The model under review builds one solid part; all positions refer to its coordinate system, in mm. Coordinates: 2 decimals unless noted, no trailing zeros. Order: outer loops, then holes, each group sorted by start corner. A loop starts at its lowest first (then second) coordinate and runs counter-clockwise, first axis right, second up. Notation, with made-up numbers: (-23, -0.75) - (-7, -0.75) arc R11 ccw to (-7, 8.25) - close; hole circle Ø4 at (-10, 31). An arc over 180 degrees is marked (long way). Answer in a Markdown table with one row per item.
```python
from build123d import *

# Parameters (mm, degrees)
F0_W     = 54
F0_H     = 48
F0_R     = 1.5
F1_DEPTH = 3
F2_R     = 1.5
F3_DEPTH = 2


with BuildPart() as f1:
    # F0 (on Front) → F1 (new body)
    with BuildSketch(Plane.XZ):
        Rectangle(F0_W, F0_H)
        with Locations((-23, -20)):
            Circle(F0_R, mode=Mode.SUBTRACT)
        with Locations((-18, -15)):
            Circle(F0_R, mode=Mode.SUBTRACT)
        with Locations((23, -20)):
            Circle(F0_R, mode=Mode.SUBTRACT)
        with Locations((18, -15)):
            Circle(F0_R, mode=Mode.SUBTRACT)
        with Locations((-18, 15)):
            Circle(F0_R, mode=Mode.SUBTRACT)
        with Locations((-23, 20)):
            Circle(F0_R, mode=Mode.SUBTRACT)
        with Locations((18, 15)):
            Circle(F0_R, mode=Mode.SUBTRACT)
        with Locations((23, 20)):
            Circle(F0_R, mode=Mode.SUBTRACT)
    extrude(amount=F1_DEPTH)

    # F2 (on face) → F3 (cut)
    with BuildSketch(Plane.XZ.offset(3)):
        Polygon((-25.6, -18.498889), (-25.6, -21.501111), (-23, -23.002221), (-20.4, -21.501111), (-20.4, -18.498889), (-23, -16.997779), align=None)
        with Locations((-23, -20)):
            Circle(F2_R, mode=Mode.SUBTRACT)
        Polygon((23, -16.997779), (20.4, -18.498889), (20.4, -21.501111), (23, -23.002221), (25.6, -21.501111), (25.6, -18.498889), align=None)
        with Locations((23, -20)):
            Circle(F2_R, mode=Mode.SUBTRACT)
        Polygon((-25.6, 21.501111), (-25.6, 18.498889), (-23, 16.997779), (-20.4, 18.498889), (-20.4, 21.501111), (-23, 23.002221), align=None)
        with Locations((-23, 20)):
            Circle(F2_R, mode=Mode.SUBTRACT)
        Polygon((20.4, 18.498889), (23, 16.997779), (25.6, 18.498889), (25.6, 21.501111), (23, 23.002221), (20.4, 21.501111), align=None)
        with Locations((23, 20)):
            Circle(F2_R, mode=Mode.SUBTRACT)
    extrude(amount=-F3_DEPTH, mode=Mode.SUBTRACT)


solid = f1.part
```
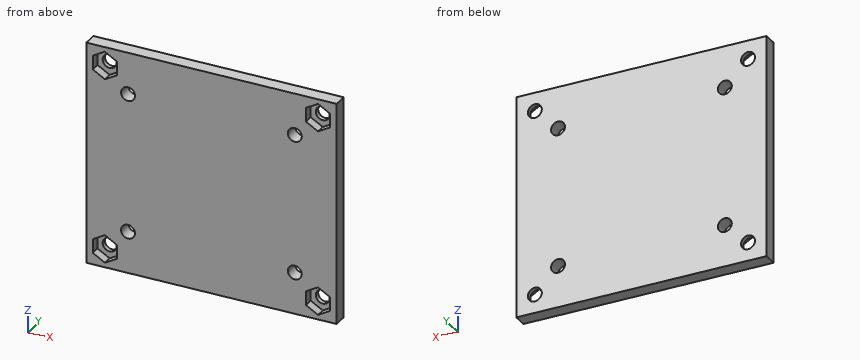
Item 1: We need section D-D, the plane z = 20. Write out the cut boundary in (x, y), then the cut area to 3 significant figures.
Check values:
| item | result |
|---|---|
| outline | (-27, -3) - (-25.6, -3) - (-25.6, -1) - (-24.5, -1) - (-24.5, 0) - (-27, 0) - close; (-21.5, -1) - (-20.4, -1) - (-20.4, -3) - (20.4, -3) - (20.4, -1) - (21.5, -1) - (21.5, 0) - (-21.5, 0) - close; (24.5, -1) - (25.6, -1) - (25.6, -3) - (27, -3) - (27, 0) - (24.5, 0) - close |
| area | 135 mm^2 |
Item 2: To check wall thickness, follow line 1 (Z direction, x = 18, y = -1.2); line 2 (Z direction, x = 23, y = -0.15); line 3 (X direction, y = -2.4, z = -14.5). State the ranges of each line that lie inside material, in increasing order. Write a range as from..to.
Check values:
| item | result |
|---|---|
| line 1 | -24..-16.5, -13.5..13.5, 16.5..24 |
| line 2 | -24..-21.5, -18.5..18.5, 21.5..24 |
| line 3 | -27..-19.41, -16.59..16.59, 19.41..27 |
Item 3: We need section B-B, the plane x = 18. Write out the cut boundary in (y, z), then the cut area to 3 significant figures.
Check values:
| item | result |
|---|---|
| outline | (-3, -24) - (0, -24) - (0, -16.5) - (-3, -16.5) - close; (-3, -13.5) - (0, -13.5) - (0, 13.5) - (-3, 13.5) - close; (-3, 16.5) - (0, 16.5) - (0, 24) - (-3, 24) - close |
| area | 126 mm^2 |
Item 4: Clearance check with flat-ended pins moving along their axes: pin 1 Ø3.5 at (x, z) = (-18, 15) entering from +Y; pin 2 Ø3.5 at (x, z) = (-23, 20) entering from -Y. State where each tip first meets the part, or that it passes through.
Check values:
| item | result |
|---|---|
| pin 1 | y = 0 |
| pin 2 | y = -1 |
Item 5: We need section C-C, the plane y = -2.45. State how many separate pieces and enclosed holes the cut face has, then the cut area to 3 significant figures.
Check values:
| item | result |
|---|---|
| separate pieces | 1 |
| enclosed holes | 8 |
| area | 2,470 mm^2 |
Item 6: We need section A-A, the plane z = 15. Write out the cut boundary in (x, y), then the cut area to 3 significant figures.
Check values:
| item | result |
|---|---|
| outline | (-27, -3) - (-19.5, -3) - (-19.5, 0) - (-27, 0) - close; (-16.5, -3) - (16.5, -3) - (16.5, 0) - (-16.5, 0) - close; (19.5, -3) - (27, -3) - (27, 0) - (19.5, 0) - close |
| area | 144 mm^2 |
